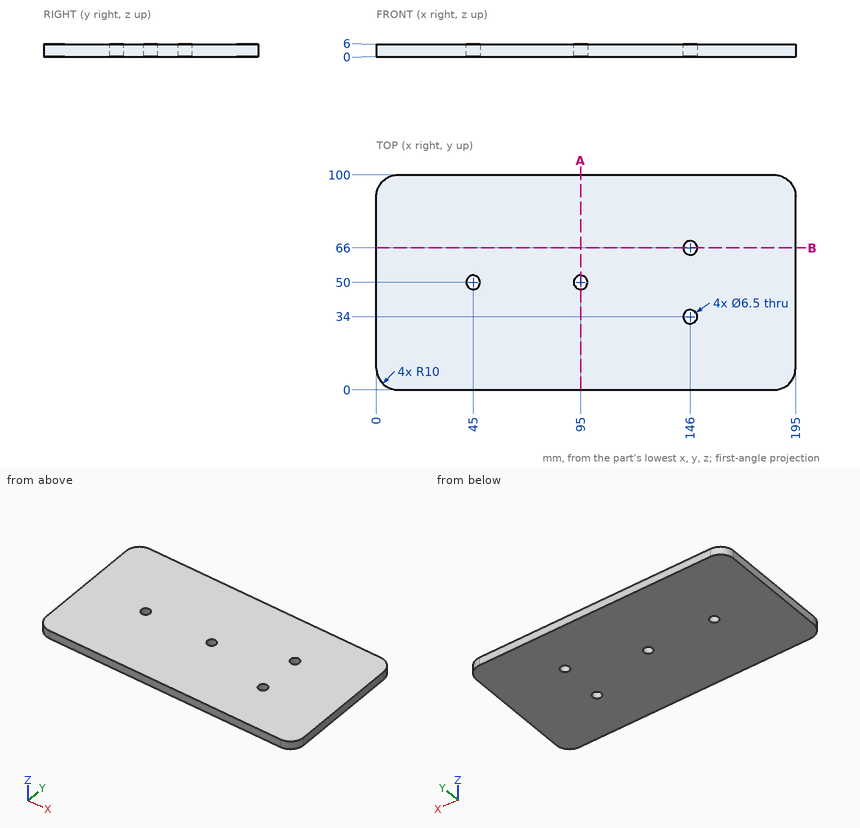
Answer from the drawing. Dimensions are ordinates in mm from the lowest x, y and z of the part. Round coordinates to 2 decimals unless told otherwise and drop trailing zeros. Write each loop counter-clockwise with the first axis right and the second up, starting at its lowest first coordinate (ties: lowest second). Pieces come first, ordered by that corner, then holes. Notation, with made-up numbers: M -26,9.5 L 0,9.5 A8 cw 0,17.5 Z; hole C 88.5,-10 d8. An arc over 180 degrees is marked long. Write each question's results on one line, items separated by ' | '. Start each with the question number.
Item 1: Given pin 1 Ø5 at (x, y) = (101.5, 48) entering from -Z, flat-ended and moving along its own axis, determine where the tip first touches the part or whether it passes through.
Item 2: Find section B-B on y = 66. Write down the section's boundary in (x, z), and give its area (3 significant figures).
Item 3: Straight lines are drawn through the part: probe 1 along Y at (x, z) = (146, 4.3); probe 2 along Y at (x, z) = (45, 1.7); probe 3 along X at (y, z) = (51, 3.9). For each, find the intervals that lie inside material, in ascending order.
Item 4: Find section A-A on x = 95. Write down the section's boundary in (y, z).
Answer block:
1) pin 1: stops at z = 0
2) outline: M 0,0 L 142.75,0 L 142.75,6 L 0,6 Z; M 149.25,0 L 195,0 L 195,6 L 149.25,6 Z | area: 1,130 mm²
3) probe 1: y = 0 to 30.75, 37.25 to 62.75, 69.25 to 100 | probe 2: y = 0 to 46.75, 53.25 to 100 | probe 3: x = 0 to 41.91, 48.09 to 91.91, 98.09 to 195
4) outline: M 0,0 L 46.75,0 L 46.75,6 L 0,6 Z; M 53.25,0 L 100,0 L 100,6 L 53.25,6 Z
